```python
from build123d import *

# Parameters (mm, degrees)
F3_DEPTH = 6.35
F1_R     = 3.175
F4_DEPTH = 9.525
F2_R     = 3.175
F5_DEPTH = 12.7
F6_R     = 0.254


with BuildPart() as f3:
    # F0 (on Front) → F3 (new body, symmetric)
    with BuildSketch(Plane.XZ):
        with BuildLine():
            Line((-8.975765, 0), (8.975765, 0))
            ThreePointArc((8.975765, 0), (0, 17.145), (-8.975765, 0))
        make_face()
    extrude(amount=F3_DEPTH, both=True)

    # F1 (on Front) → F4 (join, symmetric)
    with BuildSketch(Plane.XZ):
        with Locations((0, 6.223)):
            Circle(F1_R)
    extrude(amount=F4_DEPTH, both=True)

    # F2 (on Top) → F5 (cut)
    with BuildSketch(Plane.XY):
        Circle(F2_R)
    extrude(amount=F5_DEPTH, mode=Mode.SUBTRACT)

    # F6
    f6_edges = [f3.edges().sort_by_distance(p)[0] for p in [
        (-3.175, -9.525, 6.223),
        (0, -6.35, 17.145),
        (0, 6.35, 17.145),
        (-3.175, 9.525, 6.223),
        (0, 6.35, 0),
        (0, -6.35, 0),
    ]]
    fillet(f6_edges, radius=F6_R)


solid = f3.part
```
Can you work these out from the model? Positions are in its coordinate system, mm. A direction names the side the tool comes from. Coordinates: 2 decimals unless noted, no trailing zeros. Order: outer loops, then holes, each group sorted by start corner. A loop starts at its lowest first (then second) coordinate and runs counter-clockwise, first axis right, second up. Notation, with made-up numbers: (-18.5, 75.5) - (-3.5, 75.5) arc R19 ccw to (-3.5, 101.5) - close; hole circle Ø9 at (12, -7.75). An arc over 180 degrees is marked (long way). Answer in a Markdown table with one row per item.
1. For pin 1 (5 mm diameter, centred on x = -1.5, z = 12.5, fed in from +Y); pin 2 (4 mm diameter, centred on y = 1, z = 2, fed in from -X); pin 3 (6 mm diameter, centred on x = 6, z = 11, fed in from -Y), each with a flat end and sliding along its axis, tell me the tip position at first contact or that it passes through.
Reply:
| item | result |
|---|---|
| pin 1 | stops at y = 6.35 |
| pin 2 | stops at x = -10.69 |
| pin 3 | stops at y = -6.35 |
2. Suppose I cut it at B-B (y = 0). Please give me the cut outline in (x, z) (3 decimals).
Reply:
| item | result |
|---|---|
| outline | (-8.976, 0) - (-3.175, 0) - (-3.175, 12.7) - (3.175, 12.7) - (3.175, 0) - (8.976, 0) arc R10.922 ccw (long way) to start |
3. If we mould it in two halves opening along Y, with no side actions, what happens to faces 4 (the cylindrical face through (-0.41, 7.79, 9.37)), 5 (the cylindrical face through (-0.69, -3.1, 6.26)), 6 (the flat face through (2, 6.35, 9)), 7 (the flat face through (0, -9.525, 6))? For each: pulls with the +Y half, pulls with the -Y half, needs draft (parallel to the pull), parting line crosses it, or undercut.
Reply:
| item | result |
|---|---|
| face 4 | needs draft |
| face 5 | undercut |
| face 6 | pulls with the +Y half |
| face 7 | pulls with the -Y half |
4. Suppose I cut it at C-C (y = 7.75). Please give me the cut outline in (x, z) (3 decimals).
Reply:
| item | result |
|---|---|
| outline | circle Ø6.35 at (0, 6.223) |
5. If I drill on line 1 along Y through (x, z) = (0, 10.25) (3 decimals); line 2 along Y through (x, z) = (-1.25, 6.75) (3 decimals); line 3 along X through (y, z) = (2.5, 8.5), over which ranges is the centre line in solid material (lowest first)?
Reply:
| item | result |
|---|---|
| line 1 | y = -6.35 to -3.175, 3.175 to 6.35 |
| line 2 | y = -9.525 to -2.919, 2.919 to 9.525 |
| line 3 | x = -10.68 to -1.96, 1.96 to 10.68 |
6. Suppose I cut it at A-A (x = 0). Please give me the cut outline in (y, z) (3 decimals), and give its area (3 significant figures).
Reply:
| item | result |
|---|---|
| outline | (-9.525, 3.302) arc R0.254 ccw to (-9.271, 3.048) - (-6.35, 3.048) - (-6.35, 0.254) arc R0.254 ccw to (-6.096, 0) - (-3.175, 0) - (-3.175, 12.7) - (3.175, 12.7) - (3.175, 0) - (6.096, 0) arc R0.254 ccw to (6.35, 0.254) - (6.35, 3.048) - (9.271, 3.048) arc R0.254 ccw to (9.525, 3.302) - (9.525, 9.144) arc R0.254 ccw to (9.271, 9.398) - (6.35, 9.398) - (6.35, 16.891) arc R0.254 ccw to (6.096, 17.145) - (-6.096, 17.145) arc R0.254 ccw to (-6.35, 16.891) - (-6.35, 9.398) - (-9.271, 9.398) arc R0.254 ccw to (-9.525, 9.144) - close |
| area | 177 mm^2 |
7. For faces 1 (the flat face through (0, 0, 12.7)), 2 (the flat face through (0, 9.525, 6)), 3 (the cylindrical face through (-0.41, -7.83, 9.37)), which set-ups out of +Z, -Z, +X, -X, +Y, -Y let a thin tool reach every point of the face, with its end or its side?
Reply:
| item | result |
|---|---|
| face 1 | -Z |
| face 2 | +Z, -Z, +X, -X, +Y |
| face 3 | -Y |
